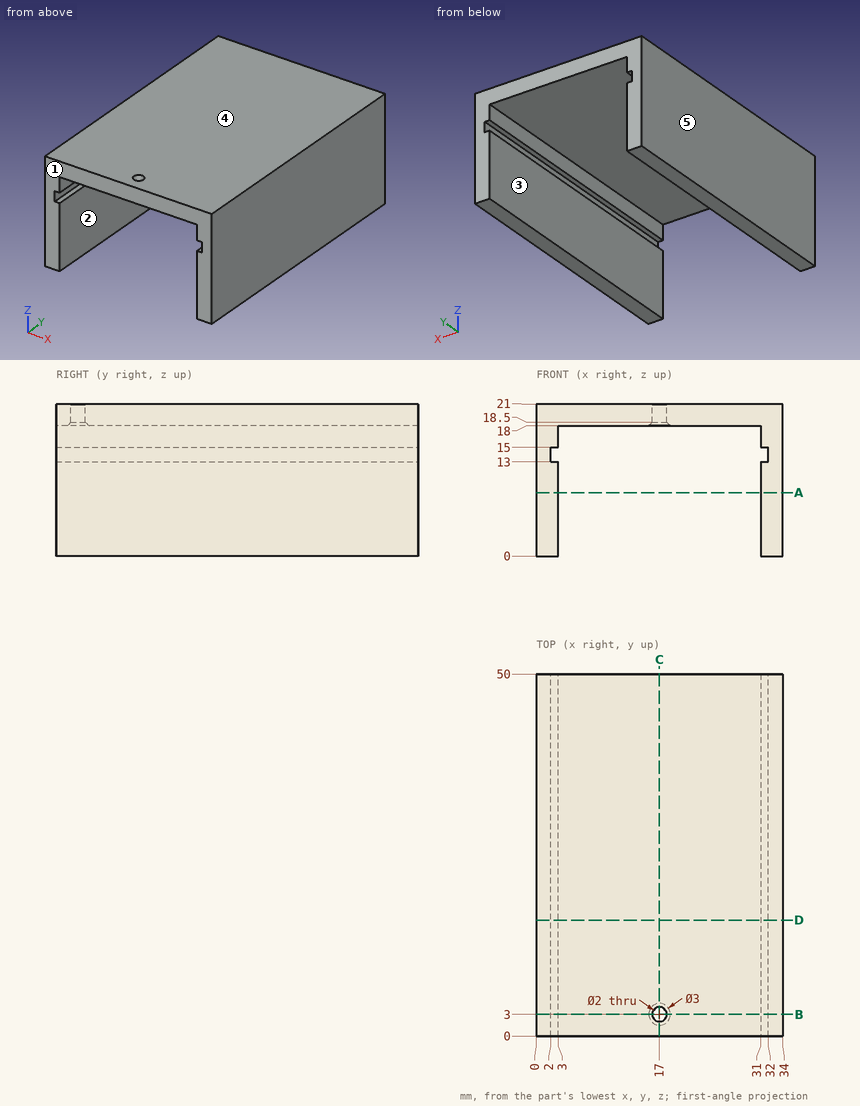
Can you work these out from the drawing? Everything is in mm from the part's minimum corner. A direction names the side the tool comes from. Coordinates: 2 decimals unless noted, no trailing zeros. Loops run counter-clockwise (first coordinate to the right, second up) from the corner with the lowest first, then second, coordinate; pieces in that order, holes last. Notation, with made-up numbers: M 32,79.5 L 72,79.5 A15 ccw 72,103.5 Z; hole C 41.25,-33.5 d8. An arc over 180 degrees is marked long. One line per item, written item: value.
1. Imagine slicing it at B-B (y = 3). List the corners of the cut face in (x, z) for me, and give its area (3 significant figures).
Geometry says:
outline: M 0,0 L 3,0 L 3,13 L 2,13 L 2,15 L 3,15 L 3,18 L 15.5,18 L 16,18.5 L 16,21 L 0,21 Z; M 18,18.5 L 18.5,18 L 31,18 L 31,15 L 32,15 L 32,13 L 31,13 L 31,0 L 34,0 L 34,21 L 18,21 Z
area: 200 mm2
2. Please list where these lines run through material, in increasing order: probe 1 along X at (y, z) = (3, 19.75); probe 2 along X at (y, z) = (27, 4.25); probe 3 along Y at (x, z) = (17, 19.75).
Geometry says:
probe 1: x = 0 to 16, 18 to 34
probe 2: x = 0 to 3, 31 to 34
probe 3: y = 0 to 2, 4 to 50
3. Imagine slicing it at D-D (y = 16). List the corners of the cut face in (x, z) for me.
Geometry says:
outline: M 0,0 L 3,0 L 3,13 L 2,13 L 2,15 L 3,15 L 3,18 L 31,18 L 31,15 L 32,15 L 32,13 L 31,13 L 31,0 L 34,0 L 34,21 L 0,21 Z
4. Will this pin go through, and if not, where does the flat tip stop? pin 1 Ø1 at (x, y) = (27.5, 16.5) entering from -Z.
Geometry says:
pin 1: stops at z = 18
5. Thinking about a two-plate mould opening in X: for the marked faces 3, 4 and 5, which applies, +X half, -X half, draft (parallel to the pull), parting line (faces both ways), or undercut?
Geometry says:
face 3: undercut
face 4: draft
face 5: -X half
6. Imagine slicing it at C-C (x = 17). List the corners of the cut face in (y, z) for me.
Geometry says:
outline: M 0,18 L 1.5,18 L 2,18.5 L 2,21 L 0,21 Z; M 4,18.5 L 4.5,18 L 50,18 L 50,21 L 4,21 Z
7. Imagine slicing it at A-A (z = 8.75). List the corners of the cut face in (x, y) for me.
Geometry says:
outline: M 0,0 L 3,0 L 3,50 L 0,50 Z; M 31,0 L 34,0 L 34,50 L 31,50 Z
8. On a 3-axis mill with a long thin cutter (end or side, diameter ignored), from which of +Z, -Z, +X, -X, +Y, -Y can I reach the whole of each face in a straight line? I mean the marked faces 1 and 2. Say none if no direction works.
Geometry says:
face 1: +Z, -Z, +X, -X, -Y
face 2: -Z, +Y, -Y
